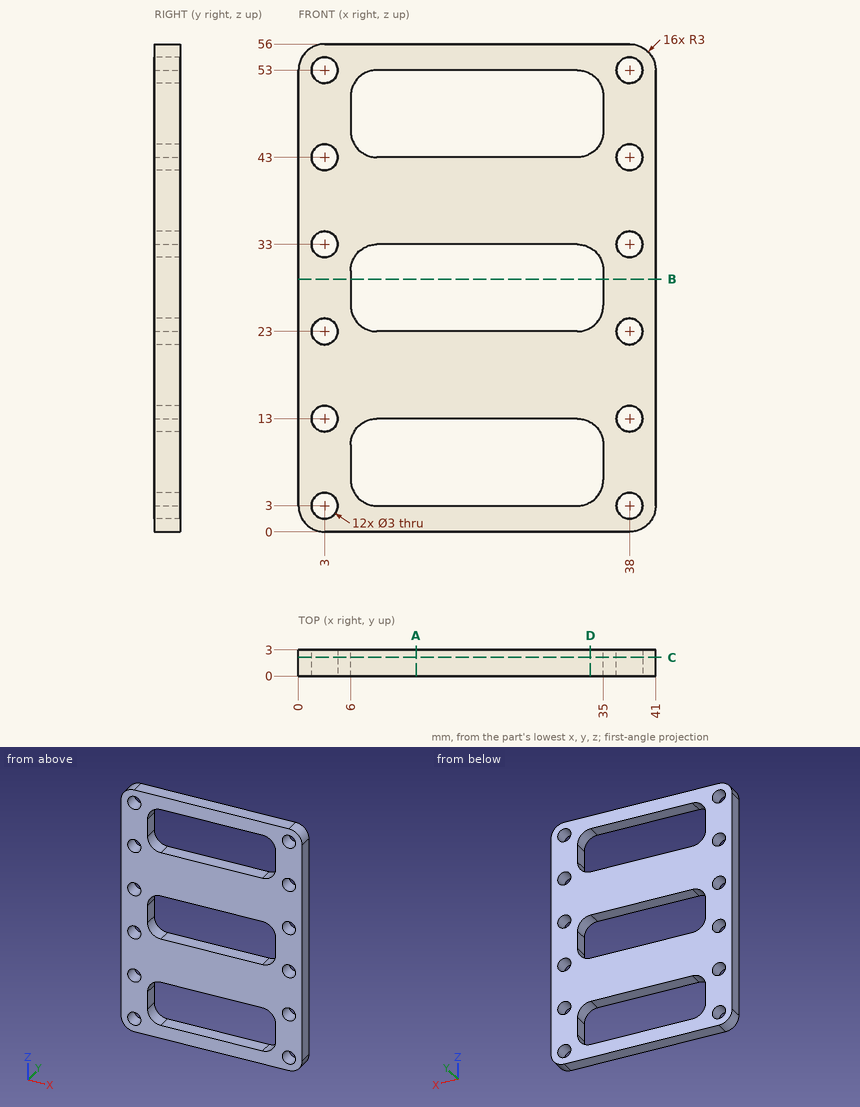
For this review, use the dimensioned drawing (mm, ordinates from the lowest corner) and the shaded views. Coordinates: 2 decimals unless noted, no trailing zeros. Order: outer loops, then holes, each group sorted by start corner. A loop starts at its lowest first (then second) coordinate and runs counter-clockwise, first axis right, second up. Notation, with made-up numbers: (38.5, -18.75) - (85.5, -18.75) arc R7 ccw to (85.5, -7.75) - close; hole circle Ø11 at (-37.75, -10). An arc over 180 degrees is marked (long way). Answer in a Markdown table with one row per item.
(1) Wall thickness on line 1 along Z through (x, y) = (24.5, 1.05); line 2 along X through (y, z) = (2.8, 12); line 3 along Z through (x, y) = (7.5, 1.7): over which ranges is each line inside the solid? List them lowest first. Write a range as from..to.
Checked values:
| item | result |
|---|---|
| line 1 | 0..3, 13..23, 33..43, 53..56 |
| line 2 | 0..1.88, 4.12..6.76, 34.24..36.88, 39.12..41 |
| line 3 | 0..3.4, 12.6..23.4, 32.6..43.4, 52.6..56 |
(2) Consider section A-A on x = 13.5. State the section outline as (y, z) points, plus the area to 3 significant figures.
Checked values:
| item | result |
|---|---|
| outline | (0, 0) - (3, 0) - (3, 3) - (0, 3) - close; (0, 13) - (3, 13) - (3, 23) - (0, 23) - close; (0, 33) - (3, 33) - (3, 43) - (0, 43) - close; (0, 53) - (3, 53) - (3, 56) - (0, 56) - close |
| area | 78.0 mm^2 |
(3) Consider section D-D on x = 33.5. State the section outline as (y, z) points.
Checked values:
| item | result |
|---|---|
| outline | (0, 0) - (3, 0) - (3, 3.4) - (0, 3.4) - close; (0, 12.6) - (3, 12.6) - (3, 23.4) - (0, 23.4) - close; (0, 32.6) - (3, 32.6) - (3, 43.4) - (0, 43.4) - close; (0, 52.6) - (3, 52.6) - (3, 56) - (0, 56) - close |
(4) Clearance check with a flat-ended pin moving along its axis: pin 1 (1.8 mm diameter, centred on x = 3, z = 3, fed in from -Y). State where the tip first meets the part, or that it passes through.
Checked values:
| item | result |
|---|---|
| pin 1 | through |
(5) Consider section B-B on z = 29. State the section outline as (x, y) points.
Checked values:
| item | result |
|---|---|
| outline | (0, 0) - (6, 0) - (6, 3) - (0, 3) - close; (35, 0) - (41, 0) - (41, 3) - (35, 3) - close |
(6) Consider section C-C on y = 2.15. Give the number of separate pieces and of enclosed holes in the cut face, plus the area to 3 significant figures.
Checked values:
| item | result |
|---|---|
| separate pieces | 1 |
| enclosed holes | 15 |
| area | 1,360 mm^2 |
